Model file for the job. Use its own axes, mm. A direction names the side the tool comes from. Give positions to 0.01 mm unless a question says otherwise; leave off trailing zeros. Order: outer loops, then holes, each group sorted by start corner. A loop starts at its lowest first (then second) coordinate and runs counter-clockwise, first axis right, second up. Notation, with made-up numbers: M 87,5.5 L 112,5.5 A33 ccw 112,40.5 Z; hole C -35.75,-6 d11. An arc over 180 degrees is marked long. Return JSON: item names as keys, results as strings. Group by question number.
1. Slice it at C-C on y = -12. List the corners of the cut face in (x, z).
2. Wall check: probe 1 along Y at (x, z) = (-23, 25); probe 2 along Z at (x, y) = (-10.5, -15.5). Give the ranges that are in metal, low to high. Write a range as [from, to].
3. Slice it at D-D on z = 16.5. List the corners of the cut face in (x, y).
4. Two-plate mould, pull along Y, no slides. Class faces 3 (the face through (-13, 0, 15)), 4 (the face through (12.124, 1, 3)), 5 (the face through (-19.22, -13.75, -9.3)): released by +Y, released by -Y, zero draft, split by the parting line, or undercut.
5. Pin check, flat tips, straight feed: pin 1 (3 mm diameter, centred on x = 3, z = 22, fed in from -Y); pin 2 (1 mm diameter, centred on x = -12.5, y = -9.5, fed in from +Z); pin 3 (12 mm diameter, centred on y = -6.5, z = 33.5, fed in from +X). Stop position of each tip, or through.
6. Slice it at B-B on x = 5.5. List the corners of the cut face in (y, z).
7. 3-axis set-ups, long thin cutter, end or side, ignore diameter. For faces 1 (the face through (-13, 1, 39.183)), 2 (the face through (-13, -16, -7.817)): which of +Z, -Z, +X, -X, +Y, -Y reach the whole face in a straight line?
8. Slice it at A-A on y = -16. List the corners of the cut face in (x, z).
from build123d import *

# Parameters (mm, degrees)
ESBO_O2_W                = 50
ESBO_O2_H                = 50
RESSALTO_EXTRUS_O1_DEPTH = 3
ESBO_O4_W                = 50
ESBO_O4_H                = 3
RESSALTO_EXTRUS_O2_DEPTH = 32
ESBO_O6_R                = 7.5
CORTE_EXTRUS_O1_DEPTH    = 69.319814067


with BuildPart() as part:
    # Esboço2 → Ressalto-extrusão1 (new body)
    with BuildSketch(Plane(origin=(0, 0, 0), x_dir=(1, 0, 0), z_dir=(0, 1, 0))):
        with Locations((-12.876074165, -14.183267942)):
            Rectangle(ESBO_O2_W, ESBO_O2_H)
    extrude(amount=RESSALTO_EXTRUS_O1_DEPTH)

    # Esboço4 → Ressalto-extrusão2 (add)
    with BuildSketch(Plane(origin=(0, 0, 0), x_dir=(-1, 0, 0), z_dir=(0, -1, 0))):
        with Locations((12.876074165, 9.316732058)):
            Rectangle(ESBO_O4_W, ESBO_O4_H)
    extrude(amount=RESSALTO_EXTRUS_O2_DEPTH)

    # Esboço6 → Corte-extrusão1 (cut, through all)
    with BuildSketch(Plane.XY.offset(-7.816732058)):
        with Locations((-26.376074165, -16)):
            Circle(ESBO_O6_R)
        with Locations((0.623925835, -16)):
            Circle(ESBO_O6_R)
    extrude(amount=-CORTE_EXTRUS_O1_DEPTH, mode=Mode.SUBTRACT)


solid = part.part
Result:
{
 "1": {"outline": "M -37.88,-10.82 L -32.72,-10.82 L -32.72,-7.82 L -37.88,-7.82 Z; M -20.03,-10.82 L -5.72,-10.82 L -5.72,-7.82 L -20.03,-7.82 Z; M 6.97,-10.82 L 12.12,-10.82 L 12.12,-7.82 L 6.97,-7.82 Z"},
 "2": {"probe 1": "y = [0, 3]", "probe 2": "z = [-10.82, -7.82]"},
 "3": {"outline": "M -37.88,0 L 12.12,0 L 12.12,3 L -37.88,3 Z"},
 "4": {"face 3": "released by -Y", "face 4": "zero draft", "face 5": "undercut"},
 "5": {"pin 1": "stops at y = 0", "pin 2": "stops at z = -7.82", "pin 3": "passes through"},
 "6": {"outline": "M -32,-10.82 L -21.7,-10.82 L -21.7,-7.82 L -32,-7.82 Z; M -10.3,-10.82 L 3,-10.82 L 3,39.18 L 0,39.18 L 0,-7.82 L -10.3,-7.82 Z"},
 "7": {"face 1": "+Z, +X, -X, +Y, -Y", "face 2": "+Z, +X, -X, -Y"},
 "8": {"outline": "M -37.88,-10.82 L -33.88,-10.82 L -33.88,-7.82 L -37.88,-7.82 Z; M -18.88,-10.82 L -6.88,-10.82 L -6.88,-7.82 L -18.88,-7.82 Z; M 8.12,-10.82 L 12.12,-10.82 L 12.12,-7.82 L 8.12,-7.82 Z"}
}
